Can you work these out from the model? Positions are in its coordinate system, mm. A direction names the side the tool comes from. Coordinates: 2 decimals unless noted, no trailing zeros. Loops run counter-clockwise (first coordinate to the right, second up) from the corner with the lowest first, then second, coordinate; pieces in that order, holes last. Notation, with made-up numbers: (41.5, 16) -> (68.5, 16) arc R19 ccw to (68.5, 48) -> close; hole circle Ø5 at (-24, 45). An arc over 180 degrees is marked (long way). Use one line per item in the form item = value. Start each with the question number.
(1) Imagine slicing it at A-A (y = 85). List the corners of the cut face in (x, z) for me.
(2) Imagine slicing it at B-B (z = 1.95). State how many separate pieces and enclosed holes the cut face has, plus the area to 3 significant figures.
(3) Imagine slicing it at D-D (x = 27.5). List the corners of the cut face in (y, z) for me, plus the area to 3 significant figures.
(4) Thinking about a two-plate mould opening in X: for faces 6 (the cylindrical face through (19.805, 86.487, 3.042)), 7 (the flat face through (-3, 20, 3)), 8 (the flat face through (25, -10, 2)), 9 (the cylindrical face through (47.39, 72.03, 4.52)), which applies, released by +X, released by -X, zero draft, split by the parting line, or undercut?
(5) I need wall thicknesses on line 1 (Y direction, x = -3, z = 1.9); line 2 (Y direction, x = -3, z = 5) (3 decimals); line 3 (X direction, y = 75, z = 1). Which ranges of each line are inside material? Lowest first, please. Write a range as [from, to].
(6) Imagine slicing it at C-C (x = -3). List the corners of the cut face in (y, z) for me (3 decimals).
(7) On a 3-axis mill with a long thin cutter (end or side, diameter ignored), from which of +Z, -Z, +X, -X, +Y, -Y can I reach the whole of each face in a straight line? I mean faces 1 (the flat face through (13, -13, 2)), 2 (the flat face through (44, 85, 3)), 3 (the cylindrical face through (44.143, 14.1, 4.521)), 4 (the flat face through (0, -5, 3)), 5 (the flat face through (44, -5, 3)). Say none if no direction works.
(8) I'm going to push flat-ended pins straight in: pin 1 (1.8 mm diameter, centred on y = 87, z = 2, fed in from +X); pin 2 (1.5 mm diameter, centred on y = -5, z = 3, fed in from -X); pin 3 (5.5 mm diameter, centred on x = -3, y = 75, fed in from +Z). Where does each tip first touch, or does it pass through?
```python
from build123d import *

# Parameters (mm, degrees)
BOSS_EXTRU_1_DEPTH      = 6
ESQUISSE2_R             = 1.5
ENL_V_MAT_EXTRU_1_DEPTH = 6
ESQUISSE6_R             = 1.5
ENL_V_MAT_EXTRU_4_DEPTH = 6
ESQUISSE7_R             = 2.995
ENL_V_MAT_EXTRU_5_DEPTH = 3
ESQUISSE8_W             = 44
ESQUISSE8_H             = 20
BOSS_EXTRU_2_DEPTH      = 6
ESQUISSE9_W             = 25
ESQUISSE9_H             = 6.5
ENL_V_MAT_EXTRU_6_DEPTH = 4
ENL_V_MAT_EXTRU_7_DEPTH = 6


with BuildPart() as part:
    # Esquisse1 → Boss.-Extru.1 (new body)
    with BuildSketch(Plane.XY):
        Polygon((-6, 70), (-6, 90), (44, 90), (44, 80), (50, 80), (50, 70), (44, 70), (44, 20), (50, 20), (50, 10), (44, 10), (44, 0), (0, 0), (0, 10), (-6, 10), (-6, 20), (0, 20), (0, 70), align=None)
    extrude(amount=BOSS_EXTRU_1_DEPTH)

    # Esquisse2 → Enlèv. mat.-Extru.1 (cut)
    with BuildSketch(Plane.XY.offset(6)):
        with Locations((20, 85)):
            Circle(ESQUISSE2_R)
    extrude(amount=-ENL_V_MAT_EXTRU_1_DEPTH, mode=Mode.SUBTRACT)

    # Esquisse6 → Enlèv. mat.-Extru.4 (cut)
    with BuildSketch(Plane.XY.offset(6)):
        with Locations((-3, 75)):
            Circle(ESQUISSE6_R)
        with Locations((-3, 15)):
            Circle(ESQUISSE6_R)
        with Locations(Location((47, 15, 0), (0, 0, 180))):
            Circle(ESQUISSE6_R)
        with Locations(Location((47, 75, 0), (0, 0, 180))):
            Circle(ESQUISSE6_R)
    extrude(amount=-ENL_V_MAT_EXTRU_4_DEPTH, mode=Mode.SUBTRACT)

    # Esquisse7 → Enlèv. mat.-Extru.5 (cut)
    with BuildSketch(Plane.XY.offset(6)):
        with Locations((-3, 15)):
            Circle(ESQUISSE7_R)
        with Locations((-3, 75)):
            Circle(ESQUISSE7_R)
        with Locations(Location((47, 75, 0), (0, 0, 180))):
            Circle(ESQUISSE7_R)
        with Locations(Location((47, 15, 0), (0, 0, 180))):
            Circle(ESQUISSE7_R)
    extrude(amount=-ENL_V_MAT_EXTRU_5_DEPTH, mode=Mode.SUBTRACT)

    # Esquisse8 → Boss.-Extru.2 (add)
    with BuildSketch(Plane(origin=(0, 0, 0), x_dir=(-1, 0, 0), z_dir=(0, 0, -1))):
        with Locations((-22, -10)):
            Rectangle(ESQUISSE8_W, ESQUISSE8_H)
    extrude(amount=-BOSS_EXTRU_2_DEPTH)

    # Esquisse9 → Enlèv. mat.-Extru.6 (cut)
    with BuildSketch(Plane(origin=(0, 0, 0), x_dir=(-1, 0, 0), z_dir=(0, 0, -1))):
        with Locations((-12.5, -9.75)):
            Rectangle(ESQUISSE9_W, ESQUISSE9_H)
    extrude(amount=-ENL_V_MAT_EXTRU_6_DEPTH, mode=Mode.SUBTRACT)

    # Esquisse10 → Enlèv. mat.-Extru.7 (cut)
    with BuildSketch(Plane(origin=(0, 0, 0), x_dir=(-1, 0, 0), z_dir=(0, 0, -1))):
        Polygon((-34, 70), (-15, -3.5), (-10, -2.207482993), (-29, 71.292517007), align=None)
    extrude(amount=-ENL_V_MAT_EXTRU_7_DEPTH, mode=Mode.SUBTRACT)


solid = part.part
```
Worked out:
q1.outline = (-6, 0) -> (18.5, 0) -> (18.5, 6) -> (-6, 6) -> close; (21.5, 0) -> (44, 0) -> (44, 6) -> (21.5, 6) -> close
q2.separate_pieces = 1
q2.enclosed_holes = 6
q2.area = 4,550 mm2
q3.outline = (-20, 0) -> (44.86, 0) -> (44.86, 6) -> (-20, 6) -> close; (65.49, 0) -> (90, 0) -> (90, 6) -> (65.49, 6) -> close
q3.area = 536 mm2
q4.face_6 = undercut
q4.face_7 = zero draft
q4.face_8 = released by -X
q4.face_9 = undercut
q5.line_1 = [10, 13.5], [16.5, 20], [70, 73.5], [76.5, 90]
q5.line_2 = [10, 12.005], [17.995, 20], [70, 72.005], [77.995, 90]
q5.line_3 = [-6, -4.5], [-1.5, 45.5], [48.5, 50]
q6.outline = (10, 0) -> (13.5, 0) -> (13.5, 3) -> (12.005, 3) -> (12.005, 6) -> (10, 6) -> close; (16.5, 0) -> (20, 0) -> (20, 6) -> (17.995, 6) -> (17.995, 3) -> (16.5, 3) -> close; (70, 0) -> (73.5, 0) -> (73.5, 3) -> (72.005, 3) -> (72.005, 6) -> (70, 6) -> close; (76.5, 0) -> (90, 0) -> (90, 6) -> (77.995, 6) -> (77.995, 3) -> (76.5, 3) -> close
q7.face_1 = -Z, -X
q7.face_2 = +Z, -Z, +X, +Y
q7.face_3 = +Z
q7.face_4 = +Z, -Z, -X, -Y
q7.face_5 = +Z, -Z, +X, -Y
q8.pin_1 = 44
q8.pin_2 = 0
q8.pin_3 = 3
